Print and shaded views of the part. All mm, measured from the part's lowest x, y and z. Coordinates: 2 decimals unless noted, no trailing zeros. Order: outer loops, then holes, each group sorted by start corner. A loop starts at its lowest first (then second) coordinate and runs counter-clockwise, first axis right, second up. Notation, with made-up numbers: (26, 2) -> (67, 2) arc R14 ccw to (67, 21) -> close; hole circle Ø2 at (80.25, 65). An arc over 180 degrees is marked (long way). Write item = value, one per line. Start each with the question number.
Q1. Cut at A-A, the plane y = 2.8. Give the number of separate pieces and of enclosed holes in the cut face, plus the area to 3 significant figures.
Q2. Cut at B-B, the plane x = 76. List the corners of the cut face in (y, z), plus the area to 4 significant figures.
Q3. Wall check: line 1 (Z direction, x = 5, y = 1.45); line 2 (Z direction, x = 54, y = 3.8); line 3 (X direction, y = 2.05, z = 60). Give the ranges that are in metal, low to high. Write a range as from..to.
Q4. Flat gauge pin, fed straight in: pin 1 (2.5 mm diameter, centred on y = 2.5, z = 63.5, fed in from -X). Where does the tip first touch, or does it go through?
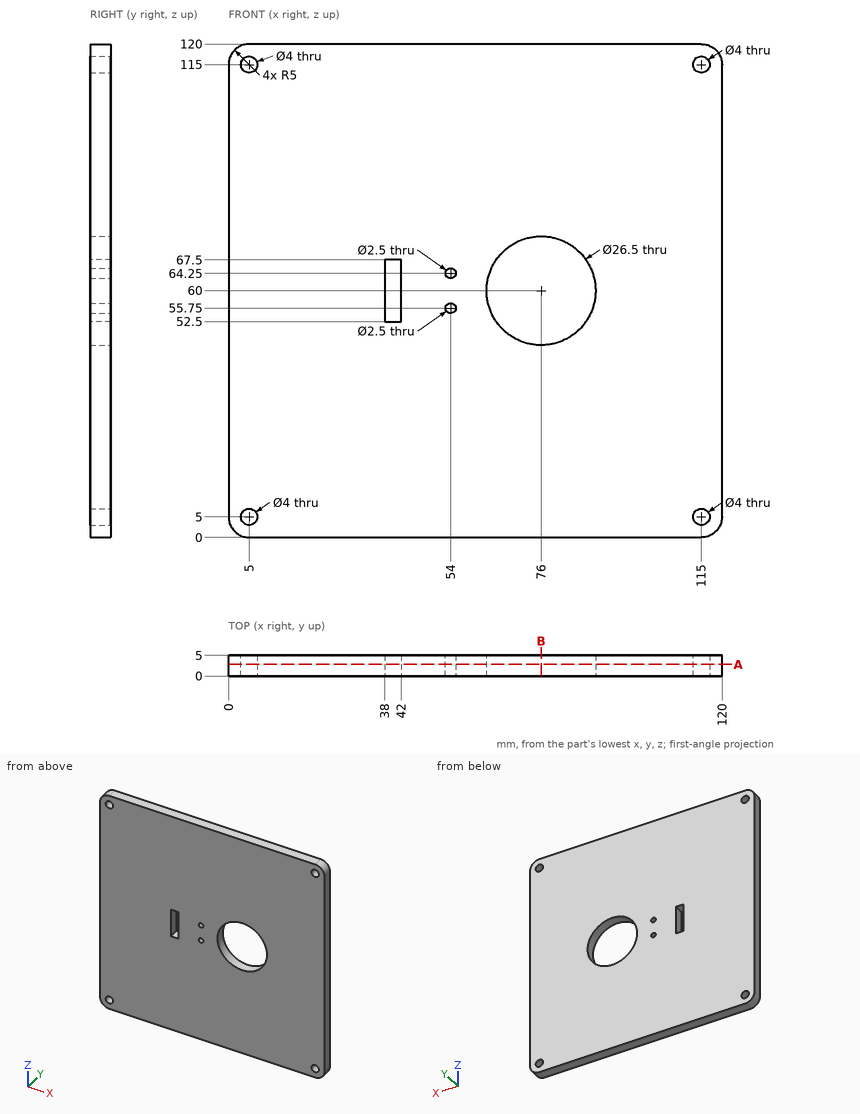
Here are the results:
q1.separate_pieces = 1
q1.enclosed_holes = 8
q1.area = 13,700 mm²
q2.outline = (0, 0) -> (5, 0) -> (5, 46.75) -> (0, 46.75) -> close; (0, 73.25) -> (5, 73.25) -> (5, 120) -> (0, 120) -> close
q2.area = 467.5 mm²
q3.line_1 = 0..3, 7..113, 117..120
q3.line_2 = 0..54.5, 57..63, 65.5..120
q3.line_3 = 0..38, 42..62.75, 89.25..120
q4.pin_1 = 0
